Can you work these out from the model? Positions are in its coordinate system, mm. A direction names the side the tool comes from. Coordinates: 2 decimals unless noted, no trailing zeros. Order: outer loops, then holes, each group sorted by start corner. A loop starts at its lowest first (then second) coordinate and runs counter-clockwise, first axis right, second up.
```python
from build123d import *

# Parameters (mm, degrees)
SKETCH_W     = 10
SKETCH_H     = 2
PAD_DEPTH    = 4
SKETCH001_W  = 25
SKETCH001_H  = 6
PAD001_DEPTH = 6
FILLET_R     = 1
FILLET001_R  = 0.2


with BuildPart() as part:
    # Sketch → Pad (new body)
    with BuildSketch(Plane.XY):
        with Locations((5, 1)):
            Rectangle(SKETCH_W, SKETCH_H)
    extrude(amount=PAD_DEPTH)

    # Sketch001 → Pad001 (join)
    with BuildSketch(Plane.XY):
        with Locations((5, 1)):
            Rectangle(SKETCH001_W, SKETCH001_H)
    extrude(amount=-PAD001_DEPTH)

    # Fillet
    fillet_edges = [part.edges().sort_by_distance(p)[0] for p in [
        (-7.5, -2, -3),
        (-7.5, 4, -3),
        (-7.5, 1, 0),
        (5, -2, 0),
        (17.5, -2, -3),
        (17.5, 1, 0),
        (5, 4, 0),
        (17.5, 4, -3),
    ]]
    fillet(fillet_edges, radius=FILLET_R)

    # Fillet001
    fillet001_edges = [part.edges().sort_by_distance(p)[0] for p in [
        (10, 0, 2),
        (10, 2, 2),
        (0, 0, 2),
        (0, 2, 2),
    ]]
    fillet(fillet001_edges, radius=FILLET001_R)


solid = part.part
```
1. Please list where these lines run through material, in increasing order: probe 1 along Y at (x, z) = (9.5, 3.75); probe 2 along Z at (x, y) = (4.75, 2.25); probe 3 along X at (y, z) = (0.95, 1.5).
Completed:
probe 1: y = 0 to 2
probe 2: z = -6 to 0
probe 3: x = 0 to 10
2. On a 3-axis mill with a long thin cutter (end or side, diameter ignored), from which of +Z, -Z, +X, -X, +Y, -Y can I reach the whole of each face in a straight line? I mean faces 1 (the flat face through (0, 1, 2)), 2 (the flat face through (10, 1, 2)), 3 (the flat face through (5, 2, 2)). Say none if no direction works.
Completed:
face 1: +Z, -X, +Y, -Y
face 2: +Z, +X, +Y, -Y
face 3: +Z, +X, -X, +Y
3. I'm going to push flat-ended pins straight in: pin 1 (1.3 mm diameter, centred on y = 1.5, z = 1.5, fed in from +X); pin 2 (3 mm diameter, centred on x = 3.5, z = 2.5, fed in from -Y); pin 3 (0.5 mm diameter, centred on y = 1.5, z = 2.5, fed in from -X). Where does each tip first touch, or does it pass through?
Completed:
pin 1: stops at x = 10
pin 2: stops at y = 0
pin 3: stops at x = 0
4. Imagine slicing it at D-D on z = -0.25. Please give me the cut outline in (x, y).
Completed:
outline: (-7.16, -1) arc R0.66 ccw to (-6.5, -1.66) - (16.5, -1.66) arc R0.66 ccw to (17.16, -1) - (17.16, 3) arc R0.66 ccw to (16.5, 3.66) - (-6.5, 3.66) arc R0.66 ccw to (-7.16, 3) - close
5. Imagine slicing it at C-C on z = 3.75. Please give me the cut outline in (x, y).
Completed:
outline: (0, 0.2) arc R0.2 ccw to (0.2, 0) - (9.8, 0) arc R0.2 ccw to (10, 0.2) - (10, 1.8) arc R0.2 ccw to (9.8, 2) - (0.2, 2) arc R0.2 ccw to (0, 1.8) - close
6. Imagine slicing it at A-A on x = 5.5. Please give me the cut outline in (y, z).
Completed:
outline: (-2, -6) - (4, -6) - (4, -1) arc R1 ccw to (3, 0) - (2, 0) - (2, 4) - (0, 4) - (0, 0) - (-1, 0) arc R1 ccw to (-2, -1) - close
7. Imagine slicing it at B-B on y = 1. Please give me the cut outline in (x, z).
Completed:
outline: (-7.5, -6) - (17.5, -6) - (17.5, -1) arc R1 ccw to (16.5, 0) - (10, 0) - (10, 4) - (0, 4) - (0, 0) - (-6.5, 0) arc R1 ccw to (-7.5, -1) - close
